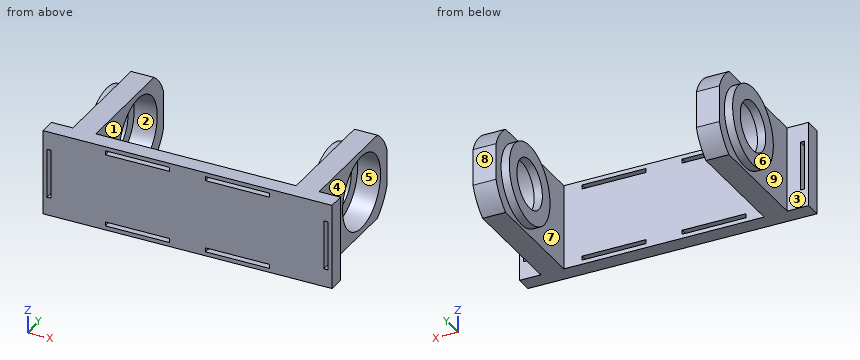
```python
from build123d import *

# Parameters (mm, degrees)
SKETCH1_W            = 20
SKETCH1_H            = 26
SKETCH1_W_2          = 1.25
SKETCH1_H_2          = 15
BOSS_EXTRUDE5_DEPTH  = 5
SKETCH3_W            = 7
SKETCH3_H            = 26
BOSS_EXTRUDE6_DEPTH  = 40
CUT_EXTRUDE1_REACH   = 55.696
SKETCH5_R            = 11.2
SKETCH6_W            = 26
SKETCH6_H            = 5
BOSS_EXTRUDE8_DEPTH  = 24
CUT_EXTRUDE2_REACH   = 102.1
SKETCH7_W            = 19.5
SKETCH7_H            = 1.25
SKETCH8_R            = 12
SKETCH8_R_2          = 7.5
BOSS_EXTRUDE9_DEPTH  = 2.5
SKETCH9_R            = 12
SKETCH9_R_2          = 7.5
BOSS_EXTRUDE10_DEPTH = 2.5


with BuildPart() as part:
    # Sketch1 → Boss-Extrude5 (new body)
    with BuildSketch(Plane(origin=(0, 0, 0), x_dir=(1, 0, 0), z_dir=(0, 1, 0))):
        with Locations((10, 13)):
            Rectangle(SKETCH1_W, SKETCH1_H)
        with Locations((1.875, 13)):
            Rectangle(SKETCH1_W_2, SKETCH1_H_2, mode=Mode.SUBTRACT)
    boss_extrude5 = extrude(amount=BOSS_EXTRUDE5_DEPTH)

    # Sketch3 → Boss-Extrude6 (add)
    with BuildSketch(Plane(origin=(0, 5, 0), x_dir=(1, 0, 0), z_dir=(0, 1, 0))):
        with Locations((10, 13)):
            Rectangle(SKETCH3_W, SKETCH3_H)
    boss_extrude6 = extrude(amount=BOSS_EXTRUDE6_DEPTH)

    # Sketch5 → Cut-Extrude1 (cut, up to next)
    with BuildSketch(Plane(origin=(13.5, 0, 0), x_dir=(0, 0, -1), z_dir=(1, 0, 0)), mode=Mode.PRIVATE) as cut_extrude1_sk1:
        with Locations((13, 30)):
            Circle(SKETCH5_R)
    cut_extrude1_tool1 = extrude(cut_extrude1_sk1.sketch, amount=-CUT_EXTRUDE1_REACH, mode=Mode.PRIVATE) & part.part
    # Sketch5 → Cut-Extrude1 (cut, up to next)
    with BuildSketch(Plane(origin=(13.5, 0, 0), x_dir=(0, 0, -1), z_dir=(1, 0, 0)), mode=Mode.PRIVATE) as cut_extrude1_sk2:
        with BuildLine():
            Line((7.432235637, 45), (0, 45))
            Line((0, 45), (0, 39.327379053))
            ThreePointArc((0, 39.327379053), (3.292522189, 42.718682107), (7.432235637, 45))
        make_face()
    cut_extrude1_tool2 = extrude(cut_extrude1_sk2.sketch, amount=-CUT_EXTRUDE1_REACH, mode=Mode.PRIVATE) & part.part
    # Sketch5 → Cut-Extrude1 (cut, up to next)
    with BuildSketch(Plane(origin=(13.5, 0, 0), x_dir=(0, 0, -1), z_dir=(1, 0, 0)), mode=Mode.PRIVATE) as cut_extrude1_sk3:
        with BuildLine():
            Line((26, 39.327379053), (26, 45))
            Line((26, 45), (18.567764363, 45))
            ThreePointArc((18.567764363, 45), (22.707477811, 42.718682107), (26, 39.327379053))
        make_face()
    cut_extrude1_tool3 = extrude(cut_extrude1_sk3.sketch, amount=-CUT_EXTRUDE1_REACH, mode=Mode.PRIVATE) & part.part
    cut_extrude1_1 = cut_extrude1_tool1.solids().sort_by_distance((13.5, 30, -13))[0]
    add(cut_extrude1_1, mode=Mode.SUBTRACT)
    cut_extrude1_2 = cut_extrude1_tool2.solids().sort_by_distance((13.5, 43.298273, -2.197768))[0]
    add(cut_extrude1_2, mode=Mode.SUBTRACT)
    cut_extrude1_3 = cut_extrude1_tool3.solids().sort_by_distance((13.5, 43.298273, -23.802232))[0]
    add(cut_extrude1_3, mode=Mode.SUBTRACT)
    cut_extrude1 = cut_extrude1_1 + cut_extrude1_2 + cut_extrude1_3  # Cut-Extrude1 as one shape, for the pattern or mirror that repeats it

    # Sketch6 → Boss-Extrude8 (add)
    with BuildSketch(Plane(origin=(20, 0, 0), x_dir=(0, 0, -1), z_dir=(1, 0, 0))):
        with Locations((13, 2.5)):
            Rectangle(SKETCH6_W, SKETCH6_H)
    boss_extrude8 = extrude(amount=BOSS_EXTRUDE8_DEPTH)

    # Mirror5: Boss-Extrude5, Boss-Extrude6, Cut-Extrude1, Boss-Extrude8 across plane
    add(boss_extrude5.mirror(Plane.ZY.offset(-44)))
    add(boss_extrude6.mirror(Plane.ZY.offset(-44)))
    add(cut_extrude1.mirror(Plane.ZY.offset(-44)), mode=Mode.SUBTRACT)
    add(boss_extrude8.mirror(Plane.ZY.offset(-44)))

    # Sketch7 → Cut-Extrude2 (cut, up to next)
    with BuildSketch(Plane(origin=(0, 5, 0), x_dir=(1, 0, 0), z_dir=(0, 1, 0)), mode=Mode.PRIVATE) as cut_extrude2_sk1:
        with Locations((28.75, 1.875)):
            Rectangle(SKETCH7_W, SKETCH7_H)
    cut_extrude2_tool1 = extrude(cut_extrude2_sk1.sketch, amount=-CUT_EXTRUDE2_REACH, mode=Mode.PRIVATE) & part.part
    # Sketch7 → Cut-Extrude2 (cut, up to next)
    with BuildSketch(Plane(origin=(0, 5, 0), x_dir=(1, 0, 0), z_dir=(0, 1, 0)), mode=Mode.PRIVATE) as cut_extrude2_sk2:
        with Locations((59.25, 1.875)):
            Rectangle(SKETCH7_W, SKETCH7_H)
    cut_extrude2_tool2 = extrude(cut_extrude2_sk2.sketch, amount=-CUT_EXTRUDE2_REACH, mode=Mode.PRIVATE) & part.part
    # Sketch7 → Cut-Extrude2 (cut, up to next)
    with BuildSketch(Plane(origin=(0, 5, 0), x_dir=(1, 0, 0), z_dir=(0, 1, 0)), mode=Mode.PRIVATE) as cut_extrude2_sk3:
        with Locations((59.25, 24.125)):
            Rectangle(SKETCH7_W, SKETCH7_H)
    cut_extrude2_tool3 = extrude(cut_extrude2_sk3.sketch, amount=-CUT_EXTRUDE2_REACH, mode=Mode.PRIVATE) & part.part
    # Sketch7 → Cut-Extrude2 (cut, up to next)
    with BuildSketch(Plane(origin=(0, 5, 0), x_dir=(1, 0, 0), z_dir=(0, 1, 0)), mode=Mode.PRIVATE) as cut_extrude2_sk4:
        with Locations((28.75, 24.125)):
            Rectangle(SKETCH7_W, SKETCH7_H)
    cut_extrude2_tool4 = extrude(cut_extrude2_sk4.sketch, amount=-CUT_EXTRUDE2_REACH, mode=Mode.PRIVATE) & part.part
    add(cut_extrude2_tool1.solids().sort_by_distance((28.75, 5, -1.875))[0], mode=Mode.SUBTRACT)
    add(cut_extrude2_tool2.solids().sort_by_distance((59.25, 5, -1.875))[0], mode=Mode.SUBTRACT)
    add(cut_extrude2_tool3.solids().sort_by_distance((59.25, 5, -24.125))[0], mode=Mode.SUBTRACT)
    add(cut_extrude2_tool4.solids().sort_by_distance((28.75, 5, -24.125))[0], mode=Mode.SUBTRACT)

    # Sketch8 → Boss-Extrude9 (add)
    with BuildSketch(Plane.ZY.offset(-6.5)):
        with Locations(Location((-13, 30, 0), (0, 0, 180))):
            Circle(SKETCH8_R)
        with Locations((-13, 30)):
            Circle(SKETCH8_R_2, mode=Mode.SUBTRACT)
    extrude(amount=BOSS_EXTRUDE9_DEPTH)

    # Sketch9 → Boss-Extrude10 (add)
    with BuildSketch(Plane.ZY.offset(-74.5)):
        with Locations(Location((-13, 30, 0), (0, 0, 180))):
            Circle(SKETCH9_R)
        with Locations((-13, 30)):
            Circle(SKETCH9_R_2, mode=Mode.SUBTRACT)
    extrude(amount=BOSS_EXTRUDE10_DEPTH)


solid = part.part
```
Geometry check sheet. Reference: the model listing, model coordinates, mm. Face numbers are marked on the shaded views. A direction names the side the tool comes from. Round coordinates to 2 decimals unless told otherwise and drop trailing zeros. Loops run counter-clockwise (first coordinate to the right, second up) from the corner with the lowest first, then second, coordinate; pieces in that order, holes last. Notation, with made-up numbers: (20, -20.5) -> (52, -20.5) arc R25 cw to (52, 16.5) -> close; hole circle Ø6 at (-35.75, 38). An arc over 180 degrees is marked (long way). Use a Markdown table: item, result.
(1) Sectioned sample at A-A (y = 30). Give the number of separate pieces and of enclosed holes in the cut face, then the cut area to 3 significant figures.
Calculated:
| item | result |
|---|---|
| separate pieces | 4 |
| enclosed holes | 0 |
| area | 95.4 mm² |
(2) Set-up check for the marked faces 1, 2, 3, 4 and 5: record each of +Z, -Z, +X, -X, +Y, -Y from which the full face is reachable in a straight line by a thin tool's end or side.
Calculated:
| item | result |
|---|---|
| face 1 | +Z, -Z, +Y |
| face 2 | none |
| face 3 | +Z, -Z, -X |
| face 4 | +Z, -Z, +X, +Y |
| face 5 | +X |
(3) Sectioned sample at B-B (x = 25). Enter the section's corners in (y, z), then the cut area to 4 significant figures.
Calculated:
| item | result |
|---|---|
| outline | (0, -26) -> (5, -26) -> (5, -24.75) -> (0, -24.75) -> close; (0, -23.5) -> (5, -23.5) -> (5, -2.5) -> (0, -2.5) -> close; (0, -1.25) -> (5, -1.25) -> (5, 0) -> (0, 0) -> close |
| area | 117.5 mm² |
(4) Sectioned sample at C-C (y = 8). Enter the section's corners in (x, z), then the cut area to 3 significant figures.
Calculated:
| item | result |
|---|---|
| outline | (6.5, -26) -> (13.5, -26) -> (13.5, 0) -> (6.5, 0) -> close; (74.5, -26) -> (81.5, -26) -> (81.5, 0) -> (74.5, 0) -> close |
| area | 364 mm² |
(5) Mould release check, pull along Y, two halves, no side actions. Record for the marked faces 6, 7, 8 and 9: released by +Y, released by -Y, zero draft, split by the parting line, or undercut.
Calculated:
| item | result |
|---|---|
| face 6 | zero draft |
| face 7 | undercut |
| face 8 | released by +Y |
| face 9 | undercut |
(6) Go/stop test with flat-tipped pins: P1, Ø6, axis at x = 32, z = -13.5, coming from the +Y side; P2, Ø8, axis at y = 34, z = -23, coming from the +X side; P3, Ø3, axis at y = 32, z = -21.5, coming from the +X side. Record where each tip stops, or that it passes through.
Calculated:
| item | result |
|---|---|
| P1 | y = 5 |
| P2 | x = 81.5 |
| P3 | x = 74.5 |
(7) Scan lines: probe 1 along X at (y, z) = (4, -17.75); probe 2 along Y at (x, z) = (72.8, -13); probe 3 along X at (y, z) = (35, -7). Record each from-to range of solid material in increasing order.
Calculated:
| item | result |
|---|---|
| probe 1 | 0 to 1.25, 2.5 to 85.5, 86.75 to 88 |
| probe 2 | 0 to 5, 18 to 22.5, 37.5 to 42 |
| probe 3 | 4 to 6.5, 72 to 74.5 |
